Geometry check sheet. Reference: drawing and pictorial views, mm from the part's lowest x, y, z. A direction names the side the tool comes from. Coordinates: 2 decimals unless noted, no trailing zeros. Write each loop counter-clockwise with the first axis right and the second up, starting at its lowest first coordinate (ties: lowest second). Pieces come first, ordered by that corner, then holes. Notation, with made-up numbers: M -16,57 L -12,57 A20 ccw -12,89 Z; hole C -27,38 d3. An arc over 180 degrees is marked long. One line per item, written item: value.
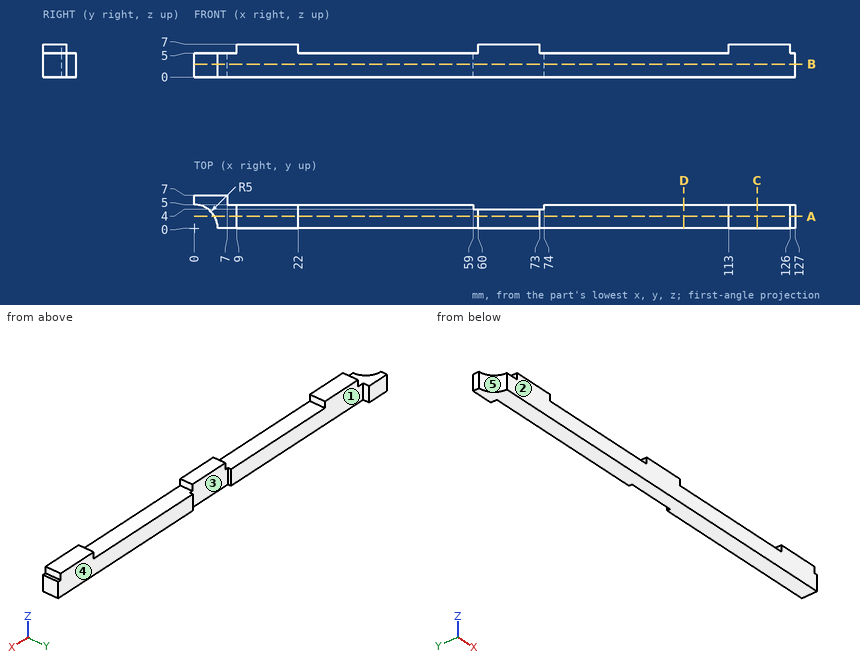
Item 1: Access from +Z, -Z, +X, -X, +Y, -Y to the whole of each face (thin tool, end or side, straight path). Record for the marked faces 1 and 2.
The answers:
face 1: +Z, -Z, +X, +Y
face 2: +Z, -Z, +X, -X, -Y
Item 2: Draft check along X on the marked faces 3, 4 and 5. Enter one of: released by +X, released by -X, zero draft, split by the parting line, or undercut.
The answers:
face 3: undercut
face 4: zero draft
face 5: released by -X
Item 3: Cross-section at A-A, the plane y = 2.5. Enter the section's corners in (x, z).
The answers:
outline: M 4.33,0 L 127,0 L 127,5 L 126,5 L 126,7 L 113,7 L 113,5 L 73,5 L 73,7 L 60,7 L 60,5 L 22,5 L 22,7 L 9,7 L 9,5 L 4.33,5 Z
Item 4: Scan lines: line 1 (X direction, y = 2.5, z = 6); line 2 (Z direction, x = 36, y = 0.5); line 3 (Y direction, x = 65, z = 4.5). Record each from-to range of solid material in increasing order.
The answers:
line 1: x = 9 to 22, 60 to 73, 113 to 126
line 2: z = 0 to 5
line 3: y = 0 to 4
Item 5: Go/stop test with flat-tipped pins: P1, Ø1.6, axis at y = 3.5, z = 6, coming from the +X side; P2, Ø1.5, axis at x = 91.5, y = 2, coming from the +Z side; P3, Ø1.5, axis at y = 1.5, z = 6, coming from the -X side; P4, Ø4, axis at x = 66, y = 4.5, coming from the -Z side. Record where each tip stops, or that it passes through.
The answers:
P1: stops at x = 126
P2: stops at z = 5
P3: stops at x = 9
P4: stops at z = 0
Item 6: Cross-section at B-B, the plane z = 2.75. Enter the section's corners in (x, y).
The answers:
outline: M 0,5 A5 cw 5,0 L 127,0 L 127,5 L 74,5 L 74,4 L 59,4 L 59,5 L 7,5 L 7,7 L 0,7 Z
Item 7: Cross-section at C-C, the plane x = 119. Enter the section's corners in (y, z).
The answers:
outline: M 0,0 L 5,0 L 5,7 L 0,7 Z
Item 8: Cross-section at D-D, the plane x = 103.5. Enter the section's corners in (y, z), and give its area (3 significant figures).
The answers:
outline: M 0,0 L 5,0 L 5,5 L 0,5 Z
area: 25.0 mm²
